Read the model definition and answer for the solid it produces. Units are mm, in the model's axes. A direction names the side the tool comes from. Coordinates: 2 decimals unless noted, no trailing zeros. Order: outer loops, then holes, each group sorted by start corner. A loop starts at its lowest first (then second) coordinate and runs counter-clockwise, first axis right, second up. Notation, with made-up numbers: (80.5, 50.25) -> (101.5, 50.25) arc R37 ccw to (101.5, 89.25) -> close; hole circle Ø8 at (-34, -6.75). An arc over 180 degrees is marked (long way). Return JSON: item names as keys, results as strings. Group by question number.
Autodesk Inventor part; units mm, degrees
ref_plane "YZ Plane" through (0, 0, 0) normal (1, 0, 0) x (0, 1, 0)
ref_plane "XZ Plane" through (0, 0, 0) normal (0, 1, 0) x (-1, 0, 0)
ref_plane "XY Plane" through (0, 0, 0) normal (0, 0, 1) x (1, 0, 0)
sketch "Sketch1" plane through (0, 0, 0) normal (0, 1, 0) x (-1, 0, 0)
  point P0 (0, 0)
sketch "Sketch2" plane through (0, 0, 0) normal (0, 1, 0) x (-1, 0, 0)
  line L0 (0, 0) -> (0, 15)
  line L1 (0, 15) -> (12, 15)
  line L2 (12, 15) -> (16.9497, 19.9497)
  line L3 (12, 15) -> (19, 15) construction
  line L4 (16.9497, 19.9497) -> (24.9497, 19.9497)
  line L5 (0, 7.5) -> (15.5, 7.5) construction
  line L6 (0, 0) -> (12, 0)
  line L7 (12, 0) -> (16.9497, -4.9497)
  line L8 (12, 0) -> (19, 0) construction
  line L9 (16.9497, -4.9497) -> (24.9497, -4.9497)
  line L10 (24.9497, 19.9497) -> (24.9497, -4.9497)
  line L11 (0, 7.5) -> (8, 7.5) construction
  circle A0 centre (8, 7.5) radius 4
  line L12 (24.9497, 7.5) -> (19.9497, 7.5) construction
  line L13 (19.9497, 7.5) -> (19.9497, 19.9497) construction
  circle A1 centre (19.9497, 13.7249) radius 2.5
  line L14 (19.9497, 7.5) -> (19.9497, -4.9497) construction
  circle A2 centre (19.9497, 1.2751) radius 2.5
  dimension "d2" = 15
  dimension "d3" = 12
  dimension "d4" = 7
  dimension "d5" = 45
  dimension "d6" = 8
  dimension "d9" = 8
  dimension "d10" = 8
  dimension "d11" = 5
  dimension "d12" = 5
extrude "Extrusion1" add sketch "Sketch2" along normal blind 3.25 contours L0 L1 L2 L4 L10 L9 L7 L6 | A0 | A1 | A2
extrude "Extrusion2" cut sketch "Sketch2" along normal blind 3.25 contours A0 | A1 | A2
properties part number "union_movllantas"
1. Given pin 1 (1 mm diameter, centred on x = -6, y = 2, fed in from -Z); pin 2 (1.5 mm diameter, centred on x = -14.5, y = 2.5, fed in from +Z); pin 3 (3 mm diameter, centred on x = -19.95, z = 1.28, fed in from -Y), each flat-ended and moving along its own axis, determine where each tip first touches the part or whether it passes through.
2. Straight lines are drawn through the part: L1, parallel to Z at x = -18, y = 3.05; L2, parallel to Z at x = -22, y = 2.4; L3, parallel to Z at x = -11.5, y = 1.6. For each, find the intervals that lie inside material, in ascending order.
3. Find section C-C on y = 0.9. Determine the outline of the cut face in (x, z), and give its area (3 significant figures).
4. Find section B-B on z = 7.5. Determine the outline of the cut face in (x, y), and give its area (3 significant figures).
5. Which of the six approach directions +Z, -Z, +X, -X, +Y, -Y give full straight-line access (tool end or side, diameter ignored) to faces 1 (the face through (-6, 2, 15)), 2 (the face through (-6, 2, 0)), 3 (the face through (-22.26, 1.6, 14.68))?
6. Find section A-A on x = -8. Determine the outline of the cut face in (y, z).
Result:
{
 "1": {"pin 1": "z = 0", "pin 2": "z = 18.25", "pin 3": "through"},
 "2": {"L1": "-4.95 to -0.29, 2.84 to 12.16, 15.29 to 19.95", "L2": "-4.95 to -0.16, 2.71 to 12.29, 15.16 to 19.95", "L3": "0 to 5.56, 9.44 to 15"},
 "3": {"outline": "(-24.95, -4.95) -> (-16.95, -4.95) -> (-12, 0) -> (0, 0) -> (0, 15) -> (-12, 15) -> (-16.95, 19.95) -> (-24.95, 19.95) -> close; hole circle Ø5 at (-19.95, 1.28); hole circle Ø5 at (-19.95, 13.72); hole circle Ø8 at (-8, 7.5)", "area": "388 mm^2"},
 "4": {"outline": "(-24.95, 0) -> (-12, 0) -> (-12, 3.25) -> (-24.95, 3.25) -> close; (-4, 0) -> (0, 0) -> (0, 3.25) -> (-4, 3.25) -> close", "area": "55.1 mm^2"},
 "5": {"face 1": "+Z, +X, +Y, -Y", "face 2": "-Z, +X, +Y, -Y", "face 3": "+Y, -Y"},
 "6": {"outline": "(0, 0) -> (3.25, 0) -> (3.25, 3.5) -> (0, 3.5) -> close; (0, 11.5) -> (3.25, 11.5) -> (3.25, 15) -> (0, 15) -> close"}
}
